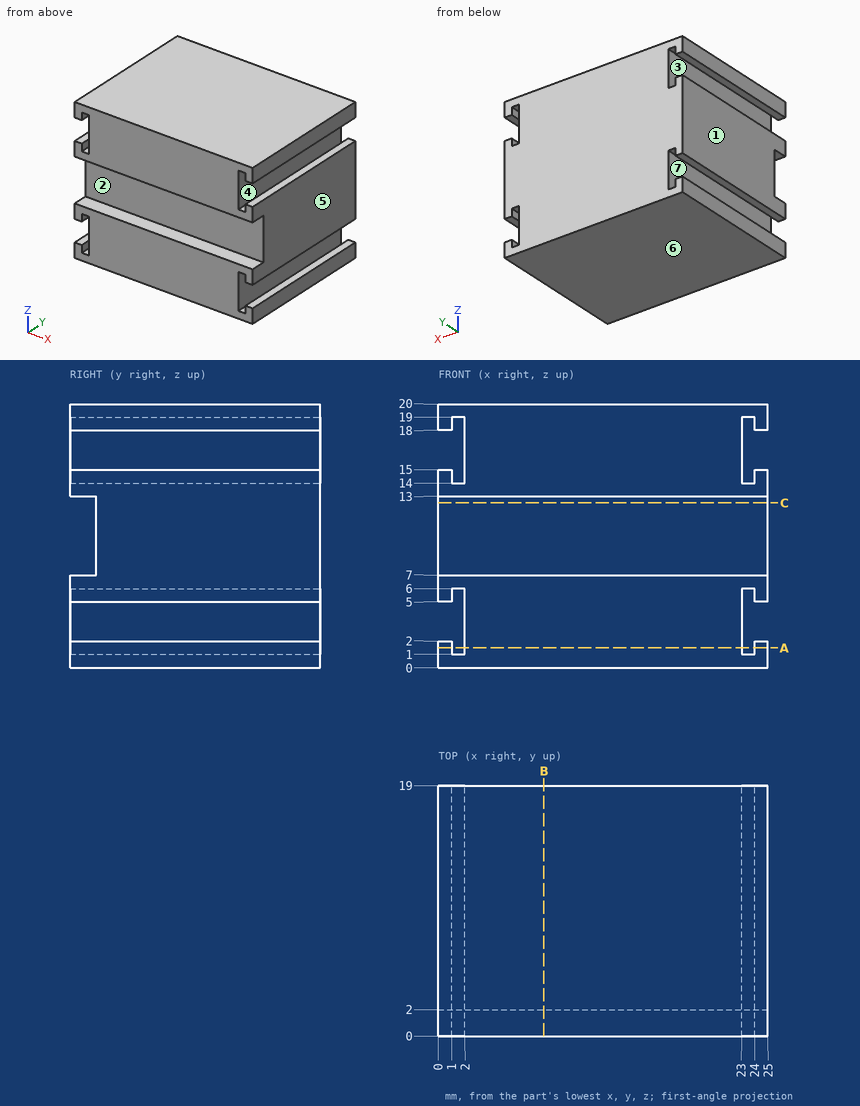
Answer from the drawing. Dimensions are ordinates in mm from the lowest x, y and z of the part. A direction names the side the tool comes from. Round coordinates to 2 decimals unless told otherwise and drop trailing zeros. Write each loop counter-clockwise with the first axis right and the second up, starting at its lowest first coordinate (ties: lowest second). Pieces come first, ordered by that corner, then holes. Notation, with made-up numbers: M 32,67 L 37,67 A9 cw 37,75 Z; hole C -26.75,-34.5 d5. An arc over 180 degrees is marked long. Write each question's results on one line, items separated by ' | '. Start each with the question number.
Item 1: For the marked faces 1, 2 and 3, determine the directions among +Z, -Z, +X, -X, +Y, -Y from which every point of the face is accessible in a straight line to the end or side of a thin tool.
Item 2: A cutting plane is placed at B-B on x = 8. Write down the section's boundary in (y, z), and give its area (3 significant figures).
Item 3: Flat-ended cylindrical pins translate along their axes: pin 1 Ø2 at (x, z) = (4.5, 11.5) entering from -Y; pin 2 Ø1.5 at (y, z) = (10.5, 16) entering from +X. Find the tip coordinate at first contact, or state that the pin passes through.
Item 4: A cutting plane is placed at A-A on z = 1.5. Write down the section's boundary in (x, y).
Item 5: Straight lines are drawn through the part: L1, parallel to X at y = 12.75, z = 18.75; L2, parallel to Z at x = 23.5, y = 1.5; L3, parallel to Z at x = 18.25, y = 1.5. For each, find the intervals that lie inside material, in ascending order. Write a range as [from, to].
Item 6: For a pull along Z with two mould halves and no side action, classify the marked faces 4, 5, 6 and 7 as pulls with the +Z half, pulls with the -Z half, needs draft (parallel to the pull), parting line crosses it, or undercut.
Item 7: A cutting plane is placed at C-C on z = 12.5. Write down the section's boundary in (x, y), and give its area (3 significant figures).
Check sheet entries:
1) face 1: +Z, -Z, -X, +Y, -Y | face 2: +X, -X, -Y | face 3: +Y, -Y
2) outline: M 0,0 L 19,0 L 19,20 L 0,20 L 0,13 L 2,13 L 2,7 L 0,7 Z | area: 368 mm²
3) pin 1: y = 2 | pin 2: x = 23
4) outline: M 0,0 L 1,0 L 1,19 L 0,19 Z; M 2,0 L 23,0 L 23,19 L 2,19 Z; M 24,0 L 25,0 L 25,19 L 24,19 Z
5) L1: [0, 1], [2, 23], [24, 25] | L2: [0, 1], [6, 7], [13, 14], [19, 20] | L3: [0, 7], [13, 20]
6) face 4: undercut | face 5: needs draft | face 6: pulls with the -Z half | face 7: undercut
7) outline: M 0,2 L 25,2 L 25,19 L 0,19 Z | area: 425 mm²
